Here's how the part is built. I have some questions about the finished solid (model axes, mm). Give positions to 0.01 mm unless a question says otherwise; leave off trailing zeros. Loops run counter-clockwise (first coordinate to the right, second up) from the corner with the lowest first, then second, coordinate; pieces in that order, holes last. Notation, with made-up numbers: (-15.75, 31) - (2.25, 31) arc R19 cw to (2.25, 35) - close; hole circle Ø3 at (14, -17.5). An arc over 180 degrees is marked (long way). Use one line per item in the form item = value.
from build123d import *

# Parameters (mm, degrees)
ESBO_O1_W                  = 4
ESBO_O1_H                  = 4
RESSALTO_EXTRUS_O1_DEPTH   = 24
CORTE_EXTRUS_O1_DEPTH      = 49.083261121
CORTE_EXTRUS_O1_DEPTH_BACK = 49.083261121
ESBO_O2_R                  = 0.85


with BuildPart() as part:
    # Esboço1 → Ressalto-extrusão1 (new, symmetric)
    with BuildSketch(Plane(origin=(0, 0, 0), x_dir=(0, 0, -1), z_dir=(1, 0, 0))):
        Rectangle(ESBO_O1_W, ESBO_O1_H)
    extrude(amount=RESSALTO_EXTRUS_O1_DEPTH, both=True)

    # Esboço2 → Corte-extrusão1 (cut, two sides: drawn at the far end of the back side and taken through both)
    with BuildSketch(Plane(origin=(24, 0, 0), x_dir=(0, 0, -1), z_dir=(1, 0, 0)).offset(-CORTE_EXTRUS_O1_DEPTH_BACK)):
        Circle(ESBO_O2_R)
    extrude(amount=CORTE_EXTRUS_O1_DEPTH + CORTE_EXTRUS_O1_DEPTH_BACK, mode=Mode.SUBTRACT)


solid = part.part
(1) Thinking about a two-plate mould opening in Y: for faces 1 (the flat face through (0, -2, 0)), 2 (the flat face through (0, 2, 0)), 3 (the cylindrical face through (-0.34, -0.83, 0.18)), which applies, pulls with the +Y half, pulls with the -Y half, needs draft (parallel to the pull), parting line crosses it, or undercut?
Geometry says:
face_1 = pulls with the -Y half
face_2 = pulls with the +Y half
face_3 = undercut
(2) If we section it at C-C (x = 17): List the corners of the cut face in (y, z) for me.
Geometry says:
outline = (-2, -2) - (2, -2) - (2, 2) - (-2, 2) - close; hole circle Ø1.7 at (0, 0)
(3) If we section it at A-A (y = 0): List the corners of the cut face in (x, z) for me.
Geometry says:
outline = (-24, -2) - (24, -2) - (24, -0.85) - (-24, -0.85) - close; (-24, 0.85) - (24, 0.85) - (24, 2) - (-24, 2) - close
(4) If I drill on probe 1 along Z at (x, y) = (-7.5, 0); probe 2 along Z at (x, y) = (0, -0.75), over which ranges is the centre line in solid material (lowest first)?
Geometry says:
probe_1 = -2 to -0.85, 0.85 to 2
probe_2 = -2 to -0.4, 0.4 to 2
